```python
from build123d import *

# Parameters (mm, degrees)
IZIM1_W                     = 100
IZIM1_H                     = 60
Y_KSEKLIK_EKSTR_ZYON1_DEPTH = 15
IZIM2_W                     = 60
IZIM2_H                     = 15
KES_EKSTR_ZYON1_DEPTH       = 5
IZIM3_R                     = 14
KES_EKSTR_ZYON2_DEPTH       = 10
IZIM4_R                     = 5
KES_EKSTR_ZYON3_DEPTH       = 16
RADYUS1_R                   = 2


with BuildPart() as part:
    # Çizim1 → Yükseklik-Ekstrüzyon1 (new body)
    with BuildSketch(Plane(origin=(0, 0, 0), x_dir=(1, 0, 0), z_dir=(0, 1, 0))):
        Rectangle(IZIM1_W, IZIM1_H)
    extrude(amount=Y_KSEKLIK_EKSTR_ZYON1_DEPTH)

    # Çizim2 → Kes-Ekstrüzyon1 (cut)
    with BuildSketch(Plane(origin=(0, 15, 0), x_dir=(1, 0, 0), z_dir=(0, 1, 0))):
        with Locations((0, 22.5)):
            Rectangle(IZIM2_W, IZIM2_H)
    extrude(amount=-KES_EKSTR_ZYON1_DEPTH, mode=Mode.SUBTRACT)

    # Çizim3 → Kes-Ekstrüzyon2 (cut)
    with BuildSketch(Plane(origin=(0, 15, 0), x_dir=(1, 0, 0), z_dir=(0, 1, 0))):
        Circle(IZIM3_R)
    extrude(amount=-KES_EKSTR_ZYON2_DEPTH, mode=Mode.SUBTRACT)

    # Çizim4 → Kes-Ekstrüzyon3 (cut, through all)
    with BuildSketch(Plane(origin=(0, 15, 0), x_dir=(1, 0, 0), z_dir=(0, 1, 0))):
        with Locations((-40, -20)):
            Circle(IZIM4_R)
        with Locations((40, -20)):
            Circle(IZIM4_R)
    extrude(amount=-KES_EKSTR_ZYON3_DEPTH, mode=Mode.SUBTRACT)

    # Radyus1
    radyus1_edges = [part.edges().sort_by_distance(p)[0] for p in [
        (30, 12.5, -15),
        (-30, 12.5, -15),
    ]]
    fillet(radyus1_edges, radius=RADYUS1_R)


solid = part.part
```
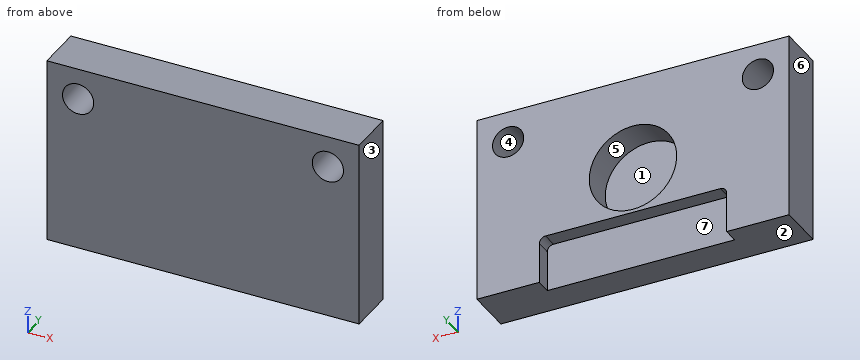
The listing builds one solid part. Answer for the finished solid, in the listing's coordinates (mm). Face numbers are marked on the shaded views. A direction names the side the tool comes from. Give positions to 0.01 mm unless a question says otherwise; leave off trailing zeros. Order: outer loops, then holes, each group sorted by start corner. A loop starts at its lowest first (then second) coordinate and runs counter-clockwise, first axis right, second up. Notation, with made-up numbers: (36, 74) - (40, 74) arc R29 ccw to (40, 111) - close; hole circle Ø8 at (20.25, -40). An arc over 180 degrees is marked (long way). Answer in a Markdown table with one row per item. Add a question column.
Q1. The part is cut by section B-B (x = -37.5). Determine the outline of the cut face in (y, z), then the cut area to 3 significant figures.
Q2. The part is cut by section A-A (y = 9). Determine the outline of the cut face in (x, z), then the cut area to 3 significant figures.
Q3. Which of the six approach directions +Z, -Z, +X, -X, +Y, -Y give full straight-line access (tool end or side, diameter ignored) to the marked faces 5, 6 and 7?
Q4. Given P1, Ø12, axis at x = -12, z = -26, coming from the +Y side, flat-ended and moving along its own axis, determine where the tip first touches the part or whether it passes through.
Q5. Find the intervals of material crossed by line 1 along X through (y, z) = (12, 20); line 2 along Z through (x, y) = (0, 9); line 3 along Z through (x, y) = (40, 3.5), in increasing order. Write a range as [from, to].
Q6. For a pull along Z with two mould halves and no side action, classify the marked faces 1, 2, 3 and 4 as released by +Z, released by -Z, zero draft, split by the parting line, or undercut.
Q7. The part is cut by section C-C (z = -9). Determine the outline of the cut face in (x, y).
Q8. The part is cut by section D-D (y = 4). Determine the outline of the cut face in (x, z).
Determined:
| question | item | result |
|---|---|---|
| 1 | outline | (0, -30) - (15, -30) - (15, 15.67) - (0, 15.67) - close; (0, 24.33) - (15, 24.33) - (15, 30) - (0, 30) - close |
| 1 | area | 770 mm² |
| 2 | outline | (-50, -30) - (50, -30) - (50, 30) - (-50, 30) - close; hole circle Ø10 at (-40, 20); hole circle Ø28 at (0, 0); hole circle Ø10 at (40, 20) |
| 2 | area | 5,230 mm² |
| 3 | face 5 | +Y |
| 3 | face 6 | +Z, -Z, -X, +Y, -Y |
| 3 | face 7 | -Z, +Y |
| 4 | P1 | stops at y = 10 |
| 5 | line 1 | x = [-50, -45], [-35, 35], [45, 50] |
| 5 | line 2 | z = [-30, -14], [14, 30] |
| 5 | line 3 | z = [-30, 15], [25, 30] |
| 6 | face 1 | undercut |
| 6 | face 2 | released by -Z |
| 6 | face 3 | zero draft |
| 6 | face 4 | undercut |
| 7 | outline | (-50, 0) - (50, 0) - (50, 15) - (10.72, 15) - (10.72, 5) - (-10.72, 5) - (-10.72, 15) - (-50, 15) - close |
| 8 | outline | (-50, -30) - (50, -30) - (50, 30) - (-50, 30) - close; hole circle Ø10 at (-40, 20); hole circle Ø10 at (40, 20) |
